```python
from build123d import *

# Parameters (mm, degrees)
SKETCH_1_R      = 23
SKETCH_1_R_2    = 20
EXTRUDE_1_DEPTH = 23
SKETCH_3_W      = 9
SKETCH_3_H      = 5
EXTRUDE_2_DEPTH = 4


with BuildPart() as part:
    # 草图1 → 凸台-拉伸1 (new body)
    with BuildSketch(Plane(origin=(0, 0, 0), x_dir=(1, 0, 0), z_dir=(0, 1, 0))):
        with Locations(Location((0, 0, 0), (0, 0, 270))):
            Circle(SKETCH_1_R)
        with Locations(Location((0, 0, 0), (0, 0, 270))):
            Circle(SKETCH_1_R_2, mode=Mode.SUBTRACT)
    extrude(amount=EXTRUDE_1_DEPTH)

    # 草图3 → 凸台-拉伸2 (add, symmetric)
    with BuildSketch(Plane.XY):
        with Locations((-26.5, 2.5)):
            Rectangle(SKETCH_3_W, SKETCH_3_H)
    extrude_2 = extrude(amount=EXTRUDE_2_DEPTH, both=True)

    # 镜向1: 凸台-拉伸2 across plane
    add(extrude_2.mirror(Plane(origin=(0, 0, 0), x_dir=(0, 0, 1), z_dir=(1, 0, 0))))


solid = part.part
```
Input: part model. Units: mm. Frame: model coordinates. A direction names the side the tool comes from. Give positions to 0.01 mm unless a question says otherwise; leave off trailing zeros. Loops run counter-clockwise (first coordinate to the right, second up) from the corner with the lowest first, then second, coordinate; pieces in that order, holes last.
1) Line query: L1, parallel to X at y = 16, z = 0; L2, parallel to Z at x = -15.5, y = 21; L3, parallel to X at y = 4.25, z = -16.5. Output: solid intervals per line, ascending.
A:
L1: x = -23 to -20, 20 to 23
L2: z = -16.99 to -12.64, 12.64 to 16.99
L3: x = -16.02 to -11.3, 11.3 to 16.02
2) Section query C-C on x = 0. Return the cut outline in (y, z), and give its area (3 significant figures).
A:
outline: (0, -23) - (23, -23) - (23, -20) - (0, -20) - close; (0, 20) - (23, 20) - (23, 23) - (0, 23) - close
area: 138 mm2
3) Section query B-B on z = 0. Return the cut outline in (x, y), and give its area (3 significant figures).
A:
outline: (-31, 0) - (-20, 0) - (-20, 23) - (-23, 23) - (-23, 5) - (-31, 5) - close; (20, 0) - (31, 0) - (31, 5) - (23, 5) - (23, 23) - (20, 23) - close
area: 218 mm2
4) Contact query for flat-ended pins moving along their axis: pin 1 (5.5 mm diameter, centred on x = 26, y = 2.5, fed in from -Z); pin 2 (2 mm diameter, centred on x = 15, y = 3, fed in from -Z); pin 3 (6.5 mm diameter, centred on x = -25, z = 1.5, fed in from +Y); pin 4 (12 mm diameter, centred on x = 19, y = 7, fed in from +Z). Output: stop coordinate, or through.
A:
pin 1: stops at z = -4
pin 2: stops at z = -18.25
pin 3: stops at y = 23
pin 4: stops at z = 18.97
5) Reachability of faces 4 (the flat face through (27, 3, -4)), 5 (the flat face through (-27, 3, -4)), 6 (the flat face through (27, 3, 4)) from +Z, -Z, +X, -X, +Y, -Y: full face, straight path, thin tool, end or side. Return the list, or none.
A:
face 4: -Z, +X, +Y, -Y
face 5: -Z, -X, +Y, -Y
face 6: +Z, +X, +Y, -Y
6) Section query D-D on x = 17.5. Return the cut outline in (y, z).
A:
outline: (0, -14.92) - (23, -14.92) - (23, -9.68) - (0, -9.68) - close; (0, 9.68) - (23, 9.68) - (23, 14.92) - (0, 14.92) - close
7) Mould query, pull axis X, two halves, no side actions, for faces 1 (the flat face through (-27, 5, 0)), 2 (the cylindrical face through (-19.524, 11.339, -4.336)), 3 (the cylindrical face through (-22.453, 11.339, -4.986)). Classes: released by +X, released by -X, zero draft, split by the parting line, or undercut.
A:
face 1: zero draft
face 2: undercut
face 3: split by the parting line
8) Section query A-A on y = 3. Return the cut outline in (x, z), and give its area (3 significant figures).
A:
outline: (-31, -4) - (-22.65, -4) arc R23 ccw to (22.65, -4) - (31, -4) - (31, 4) - (22.65, 4) arc R23 ccw to (-22.65, 4) - (-31, 4) - close; hole circle Ø40 at (0, 0)
area: 535 mm2
